Design review of the part built by this model. Coordinates are the model's own, in mm. A direction names the side the tool comes from. Give positions to 0.01 mm unless a question says otherwise; leave off trailing zeros. Loops run counter-clockwise (first coordinate to the right, second up) from the corner with the lowest first, then second, coordinate; pieces in that order, holes last. Notation, with made-up numbers: (47.25, 6.25) -> (77.25, 6.25) arc R23 cw to (77.25, 24.25) -> close; hole circle Ø2 at (60.5, 27.25). An arc over 180 degrees is marked (long way). Use a Markdown table: item, result. Add a question column.
1. For faces 4 (the cylindrical face through (-42.14, 45.58, 121.92)), 5 (the cylindrical face through (-6.503, -29.287, 98.6)), 6 (the flat face through (0, 0, 99)), list the 3-axis set-ups (+Z, -Z, +X, -X, +Y, -Y) from which the entire face can be reached by the end or side of a thin tool; tool diameter is ignored.
2. To check wall thickness, follow line 1 (X direction, y = 0, z = 44); line 2 (X direction, y = 49, z = 100.5); line 3 (Z direction, x = -38.5, y = 41.5). State the ranges of each line that lie inside material, in increasing order.
3. For pin 1 Ø11.5 at (x, z) = (37.79, 100.35) entering from +Y; pin 2 Ø5 at (x, z) = (36, 80.5) entering from -Y; pin 3 Ø13 at (x, z) = (-0.35, 137.79) entering from -Y; pin 4 Ø2 at (x, z) = (11, 131.5) entering from -Y, all flat-tipped, find the tip position at first contact; note any pin that passes through.
4. Add section D-D (y = -5). State the section outline as (x, z) points.
5. Add section A-A (x = 7.5). State the section outline as (y, z) points, and give its area (3 significant figures).
6. Add section C-C (z = 108). State the section outline as (x, y) points, and give its area (3 significant figures).
7. Draft analysis for pull direction X (two halves, no side actions). For faces 1 (the cylindrical face through (-10.3, -46.37, 98.6)), 2 (the conical face through (-0.88, 40.02, 138.48)), 3 (the flat face through (31, 1, 200)), state which applies: pulls with the +X half, pulls with the -X half, needs draft (parallel to the pull), parting line crosses it, or undercut.
8. Add section B-B (y = -25.5). State the section outline as (x, z) points, and give its area (3 significant figures).
```python
from build123d import *

# Parameters (mm, degrees)
SKETCH1_R           = 47.5
SKETCH1_R_2         = 30
BOSS_EXTRUDE1_DEPTH = 200
SKETCH2_R           = 47.5
BOSS_EXTRUDE2_DEPTH = 62.5
SKETCH3_R           = 27
CUT_EXTRUDE1_DEPTH  = 4
CIRPATTERN1_COUNT   = 4


with BuildPart() as part:
    # Sketch1 → Boss-Extrude1 (new body)
    with BuildSketch(Plane.XY):
        Circle(SKETCH1_R)
        Circle(SKETCH1_R_2, mode=Mode.SUBTRACT)
    extrude(amount=BOSS_EXTRUDE1_DEPTH)

    # Sketch2 → Boss-Extrude2 (add)
    with BuildSketch(Plane(origin=(0, 62.5, 0), x_dir=(1, 0, 0), z_dir=(0, 1, 0))):
        with Locations(Location((0, -100, 0), (0, 0, 270))):
            Circle(SKETCH2_R)
    extrude(amount=-BOSS_EXTRUDE2_DEPTH)

    # Sketch3 → Cut-Extrude1 (cut)
    with BuildSketch(Plane(origin=(0, 62.5, 0), x_dir=(1, 0, 0), z_dir=(0, 1, 0))):
        with Locations(Location((0, -100, 0), (0, 0, 270))):
            Circle(SKETCH3_R)
    extrude(amount=-CUT_EXTRUDE1_DEPTH, mode=Mode.SUBTRACT)

    # Sketch6 → Ø1.0mm Dowel Hole1 (revolve, cut)
    with BuildSketch(Plane(origin=(0.350654227, 62.5, 62.212739692), x_dir=(0, 0, 1), z_dir=(1, 0, 0))):
        Polygon((0, 0), (0, 23.004303095), (5, 20), (5, 0), align=None)
    f_1_0mm_dowel_hole1 = revolve(axis=Axis((0.350654227, 68.85, 62.212739692), (0, -1, 0)), mode=Mode.SUBTRACT)

    # CirPattern1: Ø1.0mm Dowel Hole1 ×4 about axis
    cirpattern1_axis = Axis((0, 0, 100), (0, 1, 0))
    for i in range(1, CIRPATTERN1_COUNT):
        add(f_1_0mm_dowel_hole1.rotate(cirpattern1_axis, i * 360 / CIRPATTERN1_COUNT), mode=Mode.SUBTRACT)


solid = part.part
```
Taken from the geometry:
| question | item | result |
|---|---|---|
| 1 | face 4 | +Y |
| 1 | face 5 | none |
| 1 | face 6 | +Z, -Z |
| 2 | line 1 | x = -47.5 to -30, 30 to 47.5 |
| 2 | line 2 | x = -47.5 to -42.71, -32.86 to 32.79, 42.79 to 47.5 |
| 2 | line 3 | z = 72.18 to 96.39, 102.91 to 127.82 |
| 3 | pin 1 | stops at y = 62.5 |
| 3 | pin 2 | stops at y = -33.67 |
| 3 | pin 3 | stops at y = -47.5 |
| 3 | pin 4 | stops at y = -46.44 |
| 4 | outline | (-47.24, 0) -> (-29.58, 0) -> (-29.58, 200) -> (-47.24, 200) -> close; (29.58, 0) -> (47.24, 0) -> (47.24, 200) -> (29.58, 200) -> close |
| 5 | outline | (-46.9, 0) -> (-29.05, 0) -> (-29.05, 200) -> (-46.9, 200) -> close; (0, 53.1) -> (29.05, 53.1) -> (29.05, 0) -> (46.9, 0) -> (46.9, 53.1) -> (62.5, 53.1) -> (62.5, 74.06) -> (58.5, 74.06) -> (58.5, 125.94) -> (62.5, 125.94) -> (62.5, 146.9) -> (46.9, 146.9) -> (46.9, 200) -> (29.05, 200) -> (29.05, 146.9) -> (0, 146.9) -> close |
| 5 | area | 11,100 mm^2 |
| 6 | outline | (-46.82, 8) arc R47.5 ccw (long way) to (46.82, 8) -> (46.82, 62.5) -> (25.79, 62.5) -> (25.79, 58.5) -> (-25.79, 58.5) -> (-25.79, 62.5) -> (-46.82, 62.5) -> close; hole (-30, 0) arc R30 ccw to (30, 0) -> close |
| 6 | area | 7,780 mm^2 |
| 7 | face 1 | parting line crosses it |
| 7 | face 2 | undercut |
| 7 | face 3 | needs draft |
| 8 | outline | (-40.07, 0) -> (-15.8, 0) -> (-15.8, 200) -> (-40.07, 200) -> close; (15.8, 0) -> (40.07, 0) -> (40.07, 200) -> (15.8, 200) -> close |
| 8 | area | 9,710 mm^2 |
